Autodesk Inventor part; units mm, degrees
ref_plane "YZ Plane" through (0, 0, 0) normal (1, 0, 0) x (0, 1, 0)
ref_plane "XZ Plane" through (0, 0, 0) normal (0, 1, 0) x (-1, 0, 0)
ref_plane "XY Plane" through (0, 0, 0) normal (0, 0, 1) x (1, 0, 0)
sketch "Sketch1" plane through (0, 0, 0) normal (0, 1, 0) x (-1, 0, 0)
  arc A0 (13.4296, 151.8071) -> (151.8071, 13.4296) centre (0, 0) ccw
  line L0 (151.8071, 13.4296) -> (13.4296, 151.8071)
  dimension "d0" = 304.8
  dimension "d1" = 116.84
extrude "Extrusion1" add sketch "Sketch1" along normal blind 12.7
sketch "Sketch2" plane through (0, 12.7, 0) normal (0, 1, 0) x (1, 0, 0)
  line L0 (-134.6862, 9.2408) -> (8.7197, -134.721)
  line L1 (8.7197, -134.721) -> (134.6862, -9.2408)
  line L2 (134.6862, -9.2408) -> (-8.7197, 134.721)
  line L3 (-8.7197, 134.721) -> (-134.6862, 9.2408)
  point P0 (0, 0)
  dimension "d4" = 203.2
  dimension "d5" = 177.8
  dimension "d6" = 88.9
  dimension "d7" = 101.6
extrude "Extrusion4" cut sketch "Sketch2" against normal blind 0.0025
properties part number "RockSat Plate"
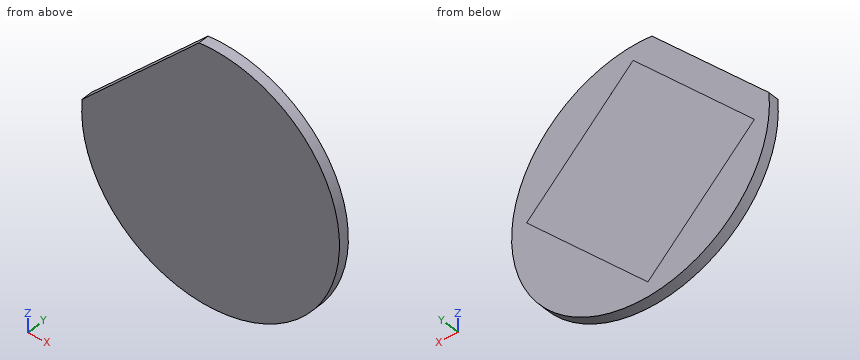
For this review, take the finished solid that the model builds, in its own axes (mm). Round coordinates to 2 decimals unless told otherwise and drop trailing zeros. Write each loop counter-clockwise with the first axis right and the second up, starting at its lowest first coordinate (ties: lowest second). Pieces come first, ordered by that corner, then holes. Notation, with made-up numbers: (-30.75, 89) - (24.25, 89) arc R18 cw to (24.25, 105) - close; hole circle Ø7 at (-7, 88.5). An arc over 180 degrees is marked (long way). Answer as a JSON object with one key per item and string values.
1. To check wall thickness, follow line 1 along Y through (x, z) = (43.5, 5.5); line 2 along Z through (x, y) = (-10.5, 8); line 3 along Z through (x, y) = (48.5, 1). State the ranges of each line that lie inside material, in increasing order.
Response values:
{"line 1": "y = 0 to 12.7", "line 2": "z = -152.04 to 152.04", "line 3": "z = -144.48 to 144.48"}
2. We need section C-C on y = 7.5. Give the boundary of the cut face in (x, z).
Response values:
{"outline": "(-151.81, 13.43) arc R152.4 ccw (long way) to (-13.43, 151.81) - close"}
3. For pin 1 Ø6 at (x, z) = (61.5, -84) entering from -Y; pin 2 Ø4 at (x, y) = (-48, 4) entering from +Z; pin 3 Ø1 at (y, z) = (5.5, -63) entering from -X; pin 4 Ø1.5 at (x, y) = (89, 8) entering from -Z, all flat-tipped, find the tip position at first contact; note any pin that passes through.
Response values:
{"pin 1": "stops at y = 0", "pin 2": "stops at z = 119.24", "pin 3": "stops at x = -138.99", "pin 4": "stops at z = -124.25"}
